Part print with two shaded views. Sizes in mm from the minimum x, y, z corner. Give positions to 0.01 mm unless a question says otherwise; leave off trailing zeros. Loops run counter-clockwise (first coordinate to the right, second up) from the corner with the lowest first, then second, coordinate; pieces in that order, holes last. Notation, with made-up numbers: M -9.5,39 L -0.5,39 A14 cw -0.5,50 Z; hole C 84.5,31.5 d9. An arc over 180 degrees is marked long. Answer in a Markdown table with one row per item.
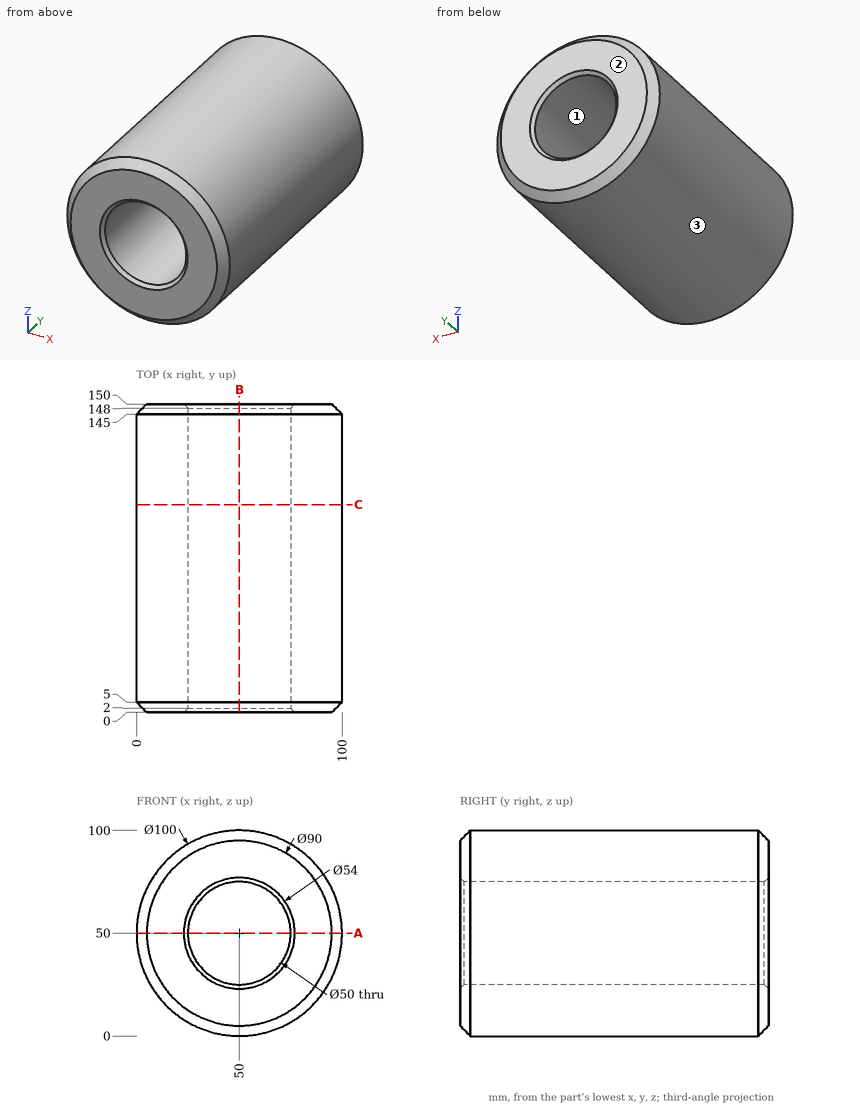
Q1. Probe probe 1 along X at (y, z) = (59, 50); probe 2 along X at (y, z) = (36.5, 31.5). List the from-to ranges inside material, lowest first.
Reported:
| item | result |
|---|---|
| probe 1 | 0 to 25, 75 to 100 |
| probe 2 | 3.55 to 33.18, 66.82 to 96.45 |
Q2. Mould opens along Z. For the marked faces 1, 2 and 3 say: released by +Z, released by -Z, zero draft, split by the parting line, or undercut.
Reported:
| item | result |
|---|---|
| face 1 | undercut |
| face 2 | zero draft |
| face 3 | split by the parting line |
Q3. Saw through at A-A (z = 50). Give the cut face in (x, y), and give its area (3 significant figures).
Reported:
| item | result |
|---|---|
| outline | M 0,5 L 5,0 L 23,0 L 25,2 L 25,148 L 23,150 L 5,150 L 0,145 Z; M 75,2 L 77,0 L 95,0 L 100,5 L 100,145 L 95,150 L 77,150 L 75,148 Z |
| area | 7,440 mm² |
Q4. Saw through at C-C (y = 101). Give the cut face in (x, z).
Reported:
| item | result |
|---|---|
| outline | C 50,50 d100; hole C 50,50 d50 |
Q5. Drop flat-ended pins along their axis: pin 1 (1.5 mm diameter, centred on y = 88, z = 62.5, fed in from +X); pin 2 (1.5 mm diameter, centred on y = 59.5, z = 76.5, fed in from +X); pin 3 (8 mm diameter, centred on y = 92.5, z = 81, fed in from -X); pin 4 (10 mm diameter, centred on x = 44, z = 34, fed in from -Y). Give the stop position or say it passes through.
Reported:
| item | result |
|---|---|
| pin 1 | x = 98.6 |
| pin 2 | x = 92.86 |
| pin 3 | x = 7.92 |
| pin 4 | through |
Q6. Saw through at B-B (x = 50). Give the cut face in (y, z), and give its area (3 significant figures).
Reported:
| item | result |
|---|---|
| outline | M 0,5 L 5,0 L 145,0 L 150,5 L 150,23 L 148,25 L 2,25 L 0,23 Z; M 0,77 L 2,75 L 148,75 L 150,77 L 150,95 L 145,100 L 5,100 L 0,95 Z |
| area | 7,440 mm² |
